Verification items for the finished model (mm, model axes). Face numbers are marked on the shaded views. A direction names the side the tool comes from. Give positions to 0.01 mm unless a question says otherwise; leave off trailing zeros. Order: outer loops, then holes, each group sorted by start corner. A loop starts at its lowest first (then second) coordinate and runs counter-clockwise, first axis right, second up.
(1) Sectioned sample at B-B on z = 18.5. Record the cut outline in (x, y), plus the area to 3 significant figures.
(2) Gauge pin test, flat ends, axial feed: pin 1 (7 mm diameter, centred on x = 0, y = 50, fed in from +Z); pin 2 (4.5 mm diameter, centred on x = 26.5, z = 15.5, fed in from +Y); pin 3 (25 mm diameter, centred on x = 11, y = 22, fed in from +Z); pin 4 (9 mm diameter, centred on x = 21.5, z = 4, fed in from +Y). Record the tip position at first contact, or that the pin passes through.
(3) Scan lines: L1, parallel to Z at x = -25, y = 3; L2, parallel to Y at x = -28, z = 13. Record each from-to range of solid material in increasing order.
(4) Mould release check, pull along Y, two halves, no side actions. Record for the marked faces 5, 6 and 7: pulls with the +Y half, pulls with the -Y half, needs draft (parallel to the pull), parting line crosses it, or undercut.
(5) Access from +Z, -Z, +X, -X, +Y, -Y to the whole of each face (thin tool, end or side, straight path). Record for the marked faces 1, 2, 3 and 4.
(6) Sectioned sample at A-A on x = 25. Record the cut outline in (y, z), plus the area to 3 significant figures.
(7) Sectioned sample at D-D on x = -21. Record the cut outline in (y, z).
(8) Sectioned sample at C-C on y = 50. Record the cut outline in (x, z), plus the area to 3 significant figures.
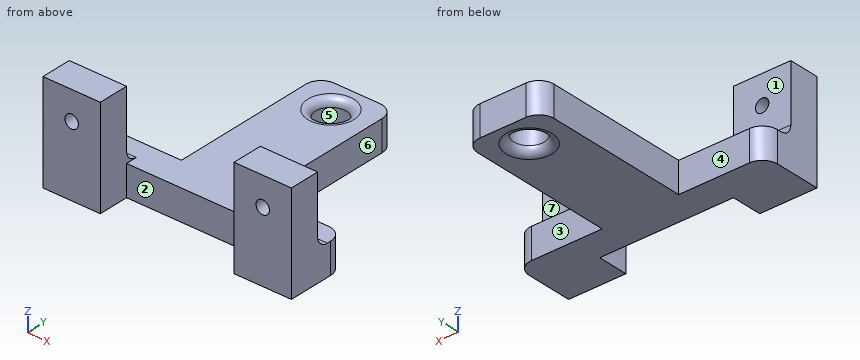
```python
from build123d import *

# Parameters (mm, degrees)
SKETCH_R     = 4
PAD_DEPTH    = 8
SKETCH001_W  = 15
SKETCH001_H  = 8
PAD001_DEPTH = 18
SKETCH002_R  = 1.75
POCKET_DEPTH = 8.001
FILLET_R     = 2
FILLET001_R  = 2
FILLET002_R  = 4
FILLET003_R  = 3


with BuildPart() as part:
    # Sketch → Pad (new body)
    with BuildSketch(Plane.XY):
        Polygon((-32.5, 0), (-17.5, 0), (-17.5, 8), (17.5, 8), (17.5, 0), (32.5, 0), (32.5, 16), (10, 16), (10, 58), (-10, 58), (-10, 16), (-32.5, 16), align=None)
        with Locations((0, 50)):
            Circle(SKETCH_R, mode=Mode.SUBTRACT)
    extrude(amount=PAD_DEPTH)

    # Sketch001 (on Face15 of Pad) → Pad001 (join)
    with BuildSketch(Plane.XY.offset(8)):
        with Locations((-25, 4)):
            Rectangle(SKETCH001_W, SKETCH001_H)
        with Locations((25, 4)):
            Rectangle(SKETCH001_W, SKETCH001_H)
    extrude(amount=PAD001_DEPTH)

    # Sketch002 (on Face11 of Pad001) → Pocket (cut, through all)
    with BuildSketch(Plane(origin=(0, 8, 0), x_dir=(-1, 0, 0), z_dir=(0, 1, 0))):
        with Locations((-25, 18.5)):
            Circle(SKETCH002_R)
        with Locations((25, 18.5)):
            Circle(SKETCH002_R)
    extrude(amount=-POCKET_DEPTH, mode=Mode.SUBTRACT)

    # Fillet
    fillet_edges = [part.edges().sort_by_distance(p)[0] for p in [
        (-4, 50, 8),
    ]]
    fillet(fillet_edges, radius=FILLET_R)

    # Fillet001
    fillet001_edges = [part.edges().sort_by_distance(p)[0] for p in [
        (-4, 50, 0),
    ]]
    fillet(fillet001_edges, radius=FILLET001_R)

    # Fillet002
    fillet002_edges = [part.edges().sort_by_distance(p)[0] for p in [
        (-10, 58, 4),
        (10, 58, 4),
        (-32.5, 16, 4),
        (32.5, 16, 4),
    ]]
    fillet(fillet002_edges, radius=FILLET002_R)

    # Fillet003
    fillet003_edges = [part.edges().sort_by_distance(p)[0] for p in [
        (25, 8, 8),
        (-25, 8, 8),
    ]]
    fillet(fillet003_edges, radius=FILLET003_R)


solid = part.part
```
Ans:
1. outline: (-32.5, 0) - (-26.75, 0) - (-26.75, 8) - (-32.5, 8) - close; (-23.25, 0) - (-17.5, 0) - (-17.5, 8) - (-23.25, 8) - close; (17.5, 0) - (23.25, 0) - (23.25, 8) - (17.5, 8) - close; (26.75, 0) - (32.5, 0) - (32.5, 8) - (26.75, 8) - close
1. area: 184 mm2
2. pin 1: passes through
2. pin 2: stops at y = 8
2. pin 3: stops at z = 8
2. pin 4: stops at y = 16
3. L1: z = 0 to 16.75, 20.25 to 26
3. L2: y = 0 to 8
4. face 5: undercut
4. face 6: needs draft
4. face 7: pulls with the +Y half
5. face 1: +Z, +X, -X, +Y
5. face 2: +Z, -Z, -Y
5. face 3: +Z, -Z, +X, +Y
5. face 4: +Z, -Z, -X, +Y
6. outline: (0, 0) - (16, 0) - (16, 8) - (11, 8) arc R3 cw to (8, 11) - (8, 16.75) - (0, 16.75) - close; (0, 20.25) - (8, 20.25) - (8, 26) - (0, 26) - close
6. area: 246 mm2
7. outline: (0, 0) - (16, 0) - (16, 8) - (11, 8) arc R3 cw to (8, 11) - (8, 26) - (0, 26) - close
8. outline: (-10, 0) - (-6, 0) arc R2 ccw to (-4, 2) - (-4, 6) arc R2 ccw to (-6, 8) - (-10, 8) - close; (4, 2) arc R2 ccw to (6, 0) - (10, 0) - (10, 8) - (6, 8) arc R2 ccw to (4, 6) - close
8. area: 92.6 mm2
